from build123d import *

# Parameters (mm, degrees)
SKETCH1_W             = 19.05
SKETCH1_H             = 6.35
SKETCH1_R             = 1.5875
BOSS_EXTRUDE1_DEPTH   = 3.175
SKETCH2_W             = 19.05
SKETCH2_H             = 9.525
BOSS_EXTRUDE2_DEPTH   = 3.175
F_8_CLEARANCE_HOLE1_D = 4.4958


with BuildPart() as part:
    # Sketch1 → Boss-Extrude1 (new body)
    with BuildSketch(Plane.XY):
        Rectangle(SKETCH1_W, SKETCH1_H)
        Circle(SKETCH1_R, mode=Mode.SUBTRACT)
    extrude(amount=BOSS_EXTRUDE1_DEPTH)

    # Sketch2 → Boss-Extrude2 (add)
    with BuildSketch(Plane.XZ.offset(3.175)):
        with Locations((0, -1.5875)):
            Rectangle(SKETCH2_W, SKETCH2_H)
    extrude(amount=BOSS_EXTRUDE2_DEPTH)

    # #8 Clearance Hole1 (through all)
    with Locations(Plane(origin=(0, -6.35, 0), x_dir=(-1, 0, 0), z_dir=(0, -1, 0))):
        with Locations((-6.35, 3.175), (6.35, 3.175)):
            Hole(F_8_CLEARANCE_HOLE1_D / 2)


solid = part.part
CAD build for the part. Positions are in the model's coordinates, mm. A direction names the side the tool comes from. Coordinates: 2 decimals unless noted, no trailing zeros. Order: outer loops, then holes, each group sorted by start corner. A loop starts at its lowest first (then second) coordinate and runs counter-clockwise, first axis right, second up. Notation, with made-up numbers: (32.5, -6) -> (71.5, -6) arc R12 ccw to (71.5, 13) -> close; hole circle Ø5 at (10.5, 80). An arc over 180 degrees is marked (long way). Answer in a Markdown table with one row per item.
1) Which spindle directions (+Z, -Z, +X, -X, +Y, -Y) get a long thin tool onto all of the face, cutting with end or side? Do faces 4 (the face through (-4.206, -4.74, -3.85)), 5 (the face through (2, 0, 0)). Say none if no direction does.
Check values:
| item | result |
|---|---|
| face 4 | +Y, -Y |
| face 5 | -Z, +X, -X, +Y |
2) Band-saw the part on B-B (y = 0). List the corners of the cut face in (x, z) (1 decimal).
Check values:
| item | result |
|---|---|
| outline | (-9.5, 0) -> (-1.6, 0) -> (-1.6, 3.2) -> (-9.5, 3.2) -> close; (1.6, 0) -> (9.5, 0) -> (9.5, 3.2) -> (1.6, 3.2) -> close |
3) Flat gauge pin, fed straight in: P1, Ø3, axis at x = 4.5, y = -1.5, coming from the -Z side. Where does the tip first touch, or does it go through?
Check values:
| item | result |
|---|---|
| P1 | z = 0 |
4) Band-saw the part on D-D (x = 6.35). List the corners of the cut face in (y, z) (3 decimals).
Check values:
| item | result |
|---|---|
| outline | (-6.35, -6.35) -> (-3.175, -6.35) -> (-3.175, -5.423) -> (-6.35, -5.423) -> close; (-6.35, -0.927) -> (-3.175, -0.927) -> (-3.175, 0) -> (3.175, 0) -> (3.175, 3.175) -> (-6.35, 3.175) -> close |
5) Drill centre lines: line 1 (Z direction, x = -6.35, y = -3.85) (3 decimals); line 2 (Y direction, x = 2.5, z = -4.25) (3 decimals); line 3 (X direction, y = -4.5, z = -2.5) (3 decimals). Where is each one in solid material? Low to high.
Check values:
| item | result |
|---|---|
| line 1 | -6.35 to -5.423, -0.927 to 3.175 |
| line 2 | -6.35 to -3.175 |
| line 3 | -9.525 to -8.494, -4.206 to 4.206, 8.494 to 9.525 |
6) Mould opens along X. For faces 1 (the face through (-9.525, -2.6, 0.5)), 2 (the face through (0, -6.35, -2)), 3 (the face through (8.494, -4.74, -3.85)) say: pulls with the +X half, pulls with the -X half, needs draft (parallel to the pull), parting line crosses it, or undercut.
Check values:
| item | result |
|---|---|
| face 1 | pulls with the -X half |
| face 2 | needs draft |
| face 3 | undercut |
